Geometry: final body of the model. Coordinates: model frame, mm. Give positions to 0.01 mm unless a question says otherwise; leave off trailing zeros. Loops run counter-clockwise (first coordinate to the right, second up) from the corner with the lowest first, then second, coordinate; pieces in that order, holes last.
1. Section B-B, the plane z = 8. Output: boundary loops of the cut face in (x, y).
2. First-contact query: P1, Ø6.5, axis at x = -46.5, z = 9, coming from the +Y side; P2, Ø5, axis at x = -39.5, z = 7, coming from the +Y side; P3, Ø1, axis at x = -39.5, y = 4, coming from the +Z side; P4, Ø3, axis at x = 19.5, z = -6, coming from the +Y side. Flat tips, straight axial feed; report the tip coordinate or a pass-through.
3. Section C-C, the plane x = 14.5. Output: boundary loops of the cut face in (y, z), then the cut area to 3 significant figures.
4. Section A-A, the plane x = -46.5. Output: boundary loops of the cut face in (y, z), then the cut area to 3 significant figures.
5. Material intervals for line 1 along X through (y, z) = (3.3, 9); line 2 along X through (y, z) = (1.7, 9); line 3 along Z through (x, y) = (39.5, 1.55), sorted ascending.
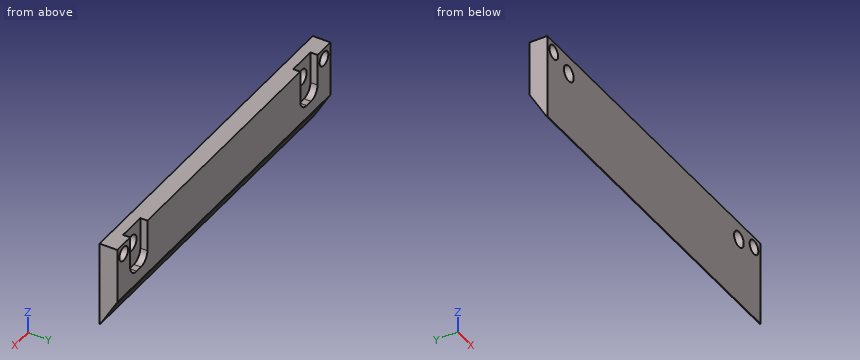
from build123d import *

# Parameters (mm, degrees)
CROQUIS1_W              = 99
CROQUIS1_H              = 24
CROQUIS1_R              = 2.017504942
CROQUIS1_R_2            = 2.25
SALIENTE_EXTRUIR1_DEPTH = 5
CORTAR_EXTRUIR1_DEPTH   = 2
CORTAR_EXTRUIR5_DEPTH   = 141


with BuildPart() as part:
    # Croquis1 → Saliente-Extruir1 (new body)
    with BuildSketch(Plane(origin=(0, 0, 0), x_dir=(1, 0, 0), z_dir=(0, 1, 0))):
        Rectangle(CROQUIS1_W, CROQUIS1_H)
        with Locations(Location((-46.5, -9, 0), (0, 0, 270))):
            Circle(CROQUIS1_R, mode=Mode.SUBTRACT)
        with Locations(Location((-39.5, -7, 0), (0, 0, 270))):
            Circle(CROQUIS1_R_2, mode=Mode.SUBTRACT)
        with Locations(Location((39.5, -7, 0), (0, 0, 270))):
            Circle(CROQUIS1_R_2, mode=Mode.SUBTRACT)
        with Locations(Location((46.5, -9, 0), (0, 0, 270))):
            Circle(CROQUIS1_R, mode=Mode.SUBTRACT)
    extrude(amount=SALIENTE_EXTRUIR1_DEPTH)

    # Croquis2 → Cortar-Extruir1 (cut)
    with BuildSketch(Plane(origin=(0, 5, 0), x_dir=(1, 0, 0), z_dir=(0, 1, 0))):
        with BuildLine():
            Line((-43.5, -3), (-43.5, -12))
            Line((-43.5, -12), (-35.5, -12))
            Line((-35.5, -12), (-35.5, -3))
            ThreePointArc((-35.5, -3), (-36.378679656, -0.878679656), (-38.5, 0))
            Line((-38.5, 0), (-40.5, 0))
            ThreePointArc((-40.5, 0), (-42.621320344, -0.878679656), (-43.5, -3))
        make_face()
        with BuildLine():
            Line((40.5, 0), (38.5, 0))
            ThreePointArc((38.5, 0), (36.378679656, -0.878679656), (35.5, -3))
            Line((35.5, -3), (35.5, -12))
            Line((35.5, -12), (43.5, -12))
            Line((43.5, -12), (43.5, -3))
            ThreePointArc((43.5, -3), (42.621320344, -0.878679656), (40.5, 0))
        make_face()
    extrude(amount=-CORTAR_EXTRUIR1_DEPTH, mode=Mode.SUBTRACT)

    # Croquis3 → Cortar-Extruir5 (cut)
    with BuildSketch(Plane.ZY.offset(49.5)):
        Polygon((-12, 5), (-12, 0.2), (-6.100895765, 3.605849418), (-3.686156124, 5), align=None)
        Polygon((-12.757171087, 0.2), (-12, 0.2), (-12, 5), (-3.686156124, 5), (-3.039853353, 5.373143079), (-12.757171087, 5.373143079), align=None)
    extrude(amount=-CORTAR_EXTRUIR5_DEPTH, mode=Mode.SUBTRACT)


solid = part.part
Answers below:
1. outline: (-49.5, 0) - (-48.25, 0) - (-48.25, 5) - (-49.5, 5) - close; (-44.75, 0) - (-41.52, 0) - (-41.52, 3) - (-43.5, 3) - (-43.5, 5) - (-44.75, 5) - close; (-37.48, 0) - (37.48, 0) - (37.48, 3) - (35.5, 3) - (35.5, 5) - (-35.5, 5) - (-35.5, 3) - (-37.48, 3) - close; (41.52, 0) - (44.75, 0) - (44.75, 5) - (43.5, 5) - (43.5, 3) - (41.52, 3) - close; (48.25, 0) - (49.5, 0) - (49.5, 5) - (48.25, 5) - close
2. P1: stops at y = 5
2. P2: stops at y = 3
2. P3: stops at z = 0
2. P4: stops at y = 4.53
3. outline: (0, -12) - (0.2, -12) - (5, -3.69) - (5, 12) - (0, 12) - close
3. area: 100 mm2
4. outline: (0, -12) - (0.2, -12) - (5, -3.69) - (5, 6.98) - (0, 6.98) - close; (0, 11.02) - (5, 11.02) - (5, 12) - (0, 12) - close
4. area: 79.9 mm2
5. line 1: x = -49.5 to -48.52, -44.48 to -43.5, -35.5 to 35.5, 43.5 to 44.48, 48.52 to 49.5
5. line 2: x = -49.5 to -48.52, -44.48 to -40.53, -38.47 to 38.47, 40.53 to 44.48, 48.52 to 49.5
5. line 3: z = -9.66 to 4.75, 9.25 to 12
